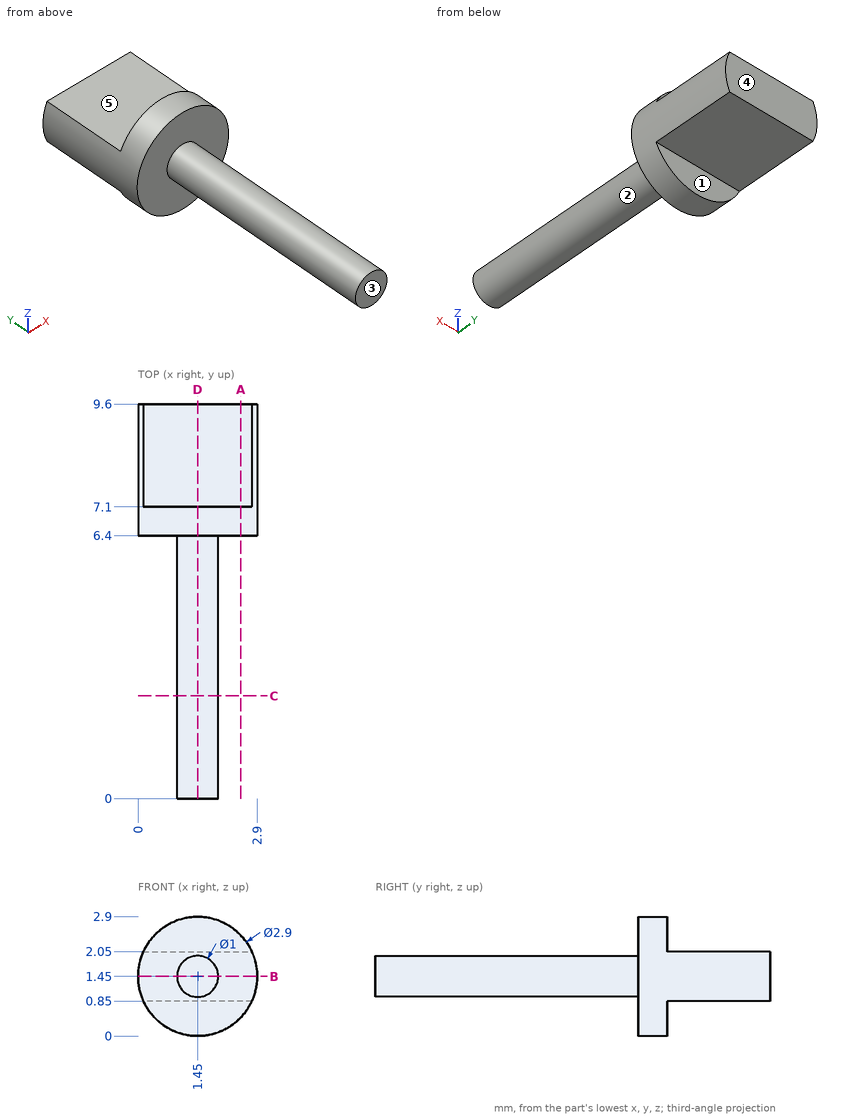
Answer from the drawing. Dimensions are ordinates in mm from the lowest x, y and z of the part. A direction names the side the tool comes from. Coordinates: 2 decimals unless noted, no trailing zeros. Write each loop counter-clockwise with the first axis right and the second up, starting at its lowest first coordinate (ties: lowest second). Pieces come first, ordered by that corner, then holes. Notation, with made-up numbers: (28.5, 7.25) - (35.5, 7.25) arc R17 cw to (35.5, 28.25) - close; hole circle Ø1 at (-1, -13). An arc over 180 degrees is marked (long way). Return JSON: item names as keys, results as strings. Group by question number.
Q1. The part is cut by section A-A on x = 2.5. Write down the section's boundary in (y, z), and give its area (3 significant figures).
Q2. Find the intervals of material crossed by line 1 along Y through (x, z) = (1.3, 2.2); line 2 along Y through (x, z) = (2.5, 1); line 3 along Z through (x, y) = (2.25, 7.25), in increasing order. Write a range as [from, to].
Q3. The part is cut by section B-B on z = 1.45. Write down the section's boundary in (x, y), and give its area (3 significant figures).
Q4. Flat-ended cylindrical pins translate along their axes: pin 1 Ø1.3 at (x, y) = (2, 9) entering from -Z; pin 2 Ø0.8 at (x, y) = (1.5, 8.5) entering from +Z; pin 3 Ø0.7 at (x, z) = (2, 2.5) entering from +Y. Find the tip coordinate at first contact, or state that the pin passes through.
Q5. The part is cut by section C-C on y = 2.5. Write down the section's boundary in (x, z), and give its area (3 significant figures).
Q6. The part is cut by section D-D on x = 1.45. Write down the section's boundary in (y, z), and give its area (3 significant figures).
Q7. Which of the six approach directions +Z, -Z, +X, -X, +Y, -Y give full straight-line access (tool end or side, diameter ignored) to the marked faces 1, 2, 3, 4 and 5?
Evaluation:
{
 "1": {"outline": "(6.4, 0.45) - (7.1, 0.45) - (7.1, 0.85) - (9.6, 0.85) - (9.6, 2.05) - (7.1, 2.05) - (7.1, 2.45) - (6.4, 2.45) - close", "area": "4.40 mm2"},
 "2": {"line 1": "y = [6.4, 7.1]", "line 2": "y = [6.4, 9.6]", "line 3": "z = [0.85, 2.05]"},
 "3": {"outline": "(0, 6.4) - (0.95, 6.4) - (0.95, 0) - (1.95, 0) - (1.95, 6.4) - (2.9, 6.4) - (2.9, 9.6) - (0, 9.6) - close", "area": "15.7 mm2"},
 "4": {"pin 1": "stops at z = 0.85", "pin 2": "stops at z = 2.05", "pin 3": "stops at y = 7.1"},
 "5": {"outline": "circle Ø1 at (1.45, 1.45)", "area": "0.785 mm2"},
 "6": {"outline": "(0, 0.95) - (6.4, 0.95) - (6.4, 0) - (7.1, 0) - (7.1, 0.85) - (9.6, 0.85) - (9.6, 2.05) - (7.1, 2.05) - (7.1, 2.9) - (6.4, 2.9) - (6.4, 1.95) - (0, 1.95) - close", "area": "11.4 mm2"},
 "7": {"face 1": "-Z, +X, -X, +Y", "face 2": "-Y", "face 3": "+Z, -Z, +X, -X, -Y", "face 4": "+Z, -Z, +X, -X, +Y", "face 5": "+Z, +X, -X, +Y"}
}
